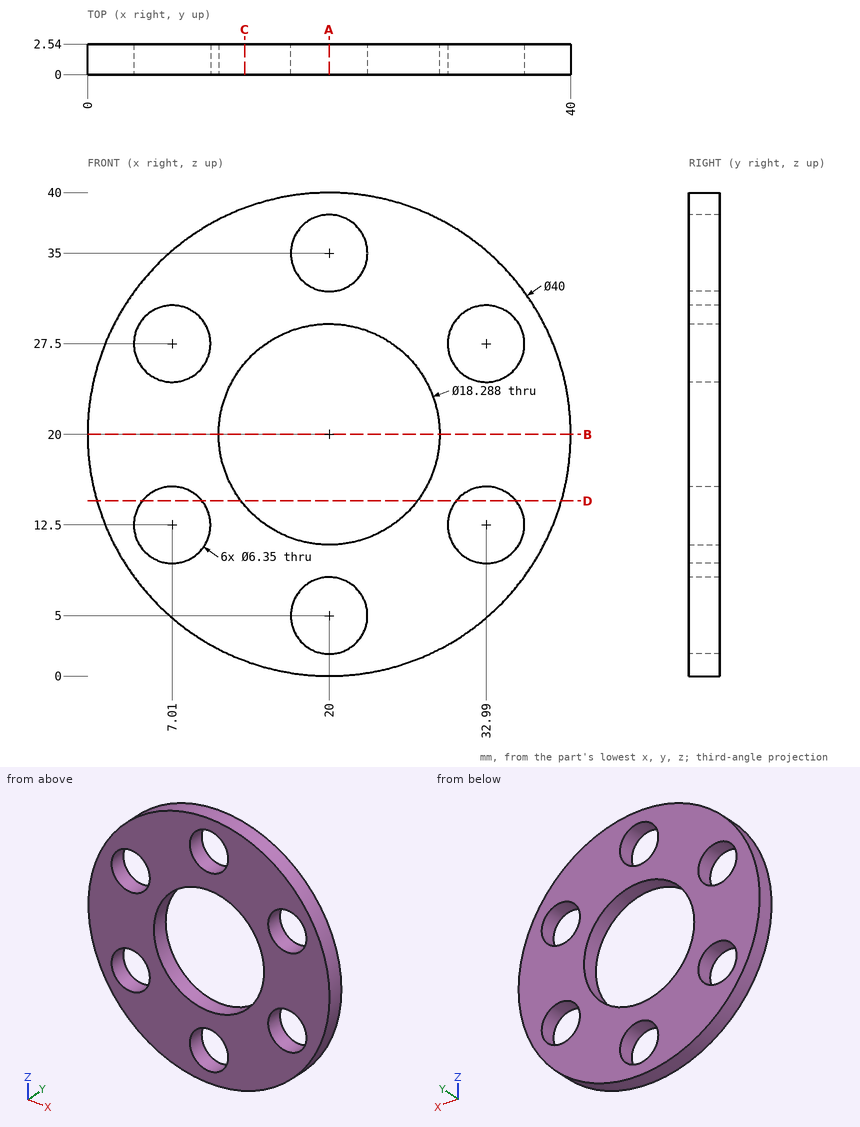
Can you work these out from the drawing? Everything is in mm from the part's minimum corner. Coordinates: 2 decimals unless noted, no trailing zeros. Write each loop counter-clockwise with the first axis right and the second up, starting at its lowest first coordinate (ties: lowest second). Pieces come first, ordered by that corner, then holes. Notation, with made-up numbers: (59, 15.5) -> (94, 15.5) arc R6 ccw to (94, 21.5) -> close; hole circle Ø11 at (-11, 58). An arc over 180 degrees is marked (long way). Write each question's results on one line, items separated by ' | '. Start each with the question number.
Q1. Imagine slicing it at A-A (x = 20). Write out the boundary of the cut face in (y, z) (1 decimal), then the cut area to 3 significant figures.
Q2. Imagine slicing it at C-C (x = 13). Write out the boundary of the cut face in (y, z) (1 decimal).
Q3. Imagine slicing it at D-D (z = 14.5). Write out the boundary of the cut face in (x, y) (1 decimal).
Q4. Imagine slicing it at B-B (z = 20). Write out the boundary of the cut face in (x, y).
Q5. I'm going to push flat-ended pins straight in: pin 1 (5 mm diameter, centred on x = 19, z = 13, fed in from -Y); pin 2 (1.5 mm diameter, centred on x = 21, y = 2.5, fed in from +Z); pin 3 (1.5 mm diameter, centred on x = 5.5, y = 0.5, fed in from +Z) (1 decimal). Where does each tip first touch, or does it pass through?
Q6. If I drill on probe 1 along Z at (x, y) = (20, 0.75) (1 decimal); probe 2 along Z at (x, y) = (6, 1.65) (1 decimal); probe 3 along Z at (x, y) = (21.5, 0.85) (1 decimal), over which ranges is the centre line in solid material (lowest first)?
Taken from the geometry:
1) outline: (0, 0) -> (2.5, 0) -> (2.5, 1.8) -> (0, 1.8) -> close; (0, 8.2) -> (2.5, 8.2) -> (2.5, 10.9) -> (0, 10.9) -> close; (0, 29.1) -> (2.5, 29.1) -> (2.5, 31.8) -> (0, 31.8) -> close; (0, 38.2) -> (2.5, 38.2) -> (2.5, 40) -> (0, 40) -> close | area: 22.9 mm^2
2) outline: (0, 1.3) -> (2.5, 1.3) -> (2.5, 14.1) -> (0, 14.1) -> close; (0, 25.9) -> (2.5, 25.9) -> (2.5, 38.7) -> (0, 38.7) -> close
3) outline: (0.8, 0) -> (4.5, 0) -> (4.5, 2.5) -> (0.8, 2.5) -> close; (9.5, 0) -> (12.7, 0) -> (12.7, 2.5) -> (9.5, 2.5) -> close; (27.3, 0) -> (30.5, 0) -> (30.5, 2.5) -> (27.3, 2.5) -> close; (35.5, 0) -> (39.2, 0) -> (39.2, 2.5) -> (35.5, 2.5) -> close
4) outline: (0, 0) -> (10.86, 0) -> (10.86, 2.54) -> (0, 2.54) -> close; (29.14, 0) -> (40, 0) -> (40, 2.54) -> (29.14, 2.54) -> close
5) pin 1: stops at y = 0 | pin 2: stops at z = 40 | pin 3: stops at z = 34.5
6) probe 1: z = 0 to 1.8, 8.2 to 10.9, 29.1 to 31.8, 38.2 to 40 | probe 2: z = 5.7 to 9.5, 15.5 to 24.5, 30.5 to 34.3 | probe 3: z = 0.1 to 2.2, 7.8 to 11, 29 to 32.2, 37.8 to 39.9
